Autodesk Inventor part; units mm, degrees
ref_plane "YZ Plane" through (0, 0, 0) normal (1, 0, 0) x (0, 1, 0)
ref_plane "XZ Plane" through (0, 0, 0) normal (0, 1, 0) x (-1, 0, 0)
ref_plane "XY Plane" through (0, 0, 0) normal (0, 0, 1) x (1, 0, 0)
sketch "Sketch1" plane through (0, 0, 0) normal (0, 0, 1) x (1, 0, 0)
  circle A0 centre (0, 0) radius 15.748
  circle A1 centre (152.4, 0) radius 15.748
  line L0 (0, 0) -> (152.4, 0)
  line L1 (0, 15.748) -> (0, -15.748)
  line L2 (152.4, 15.748) -> (152.4, -15.748)
  dimension "d2" = 15.748
  dimension "d4" = 152.4
revolve "Revolution1" add sketch "Sketch1" angle 360 about axis through (0, 15.748, 0) along (0, -1, 0) contours L1 A0
revolve "Revolution2" add sketch "Sketch1" angle 360 about axis through (152.4, 15.748, 0) along (0, -1, 0) contours A1 L2 L0 | L0 L2 A1
sketch "Sketch2" plane through (0, 0, 0) normal (1, 0, 0) x (0, 1, 0)
  circle A0 centre (0, 0) radius 6.35
  dimension "d7" = 12.7
sweep "Sweep1" add profiles "Sketch2" path "Sketch1" path curves L0
fillet "Fillet1" radius 3.175 3 edges at (14.411, -6.35, 0) (137.989, 0, 6.35) (137.989, 0, -6.35)
properties part number "Prop_Conrod" material "Nickel-Copper Alloy 400"
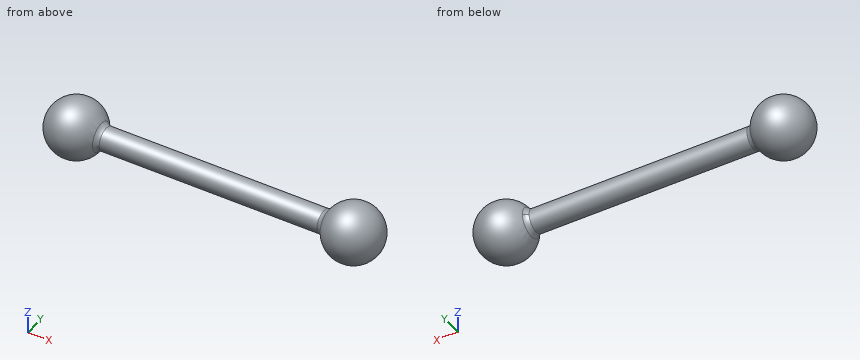
Check sheet for the modelled part. Datum: model origin and axes. Units: mm. Round coordinates to 2 decimals unless told otherwise and drop trailing zeros. Loops run counter-clockwise (first coordinate to the right, second up) from the corner with the lowest first, then second, coordinate; pieces in that order, holes last. Notation, with made-up numbers: (68.5, 89.25) -> (72.5, 89.25) arc R24 ccw to (72.5, 119.25) -> close; hole circle Ø6 at (-19.75, 41). An arc over 180 degrees is marked (long way). Answer in a Markdown table with one row per item.
Q1. Sectioned sample at A-A on z = 12. Enter the section's corners in (x, y).
Data:
| item | result |
|---|---|
| outline | circle Ø20.4 at (0, 0); circle Ø20.4 at (152.4, 0) |
Q2. Thickness scan on L1, parallel to Z at x = 51.5, y = -0.5; L2, parallel to X at y = 12.5, z = 1; L3, parallel to X at y = 4, z = 11.5. Record the ranges inside material, lowest first.
Data:
| item | result |
|---|---|
| L1 | z = -6.33 to 6.33 |
| L2 | x = -9.53 to 9.53, 142.87 to 161.93 |
| L3 | x = -9.99 to 9.99, 142.41 to 162.39 |
Q3. Sectioned sample at B-B on x = 9.5. Enter the section's corners in (y, z), then the cut area to 3 significant figures.
Data:
| item | result |
|---|---|
| outline | circle Ø25.12 at (0, 0) |
| area | 496 mm^2 |
Q4. Go/stop test with flat-tipped pins: P1, Ø10, axis at x = 113, z = 4, coming from the +Y side; P2, Ø4, axis at x = 33.5, z = -6, coming from the -Y side; P3, Ø1.5, axis at x = 5.5, z = 4, coming from the -Y side. Record where each tip stops, or that it passes through.
Data:
| item | result |
|---|---|
| P1 | stops at y = 6.35 |
| P2 | stops at y = -4.93 |
| P3 | stops at y = -14.54 |
Q5. Sectioned sample at C-C on x = 146. Enter the section's corners in (y, z), then the cut area to 3 significant figures.
Data:
| item | result |
|---|---|
| outline | circle Ø28.78 at (0, 0) |
| area | 650 mm^2 |
